```python
from build123d import *

# Parameters (mm, degrees)
SKETCH1_R             = 19.75
BOSS_EXTRUDE1_DEPTH   = 5
CUT_EXTRUDE1_DEPTH    = 4.2
F_8_CLEARANCE_HOLE1_D = 4.4958
CUT_EXTRUDE2_DEPTH    = 10


with BuildPart() as part:
    # Sketch1 → Boss-Extrude1 (new, symmetric)
    with BuildSketch(Plane(origin=(0, 0, 0), x_dir=(1, 0, 0), z_dir=(0, 1, 0))):
        with Locations(Location((0, 0, 0), (0, 0, 270))):
            Circle(SKETCH1_R)
    extrude(amount=BOSS_EXTRUDE1_DEPTH, both=True)

    # Sketch2 → Cut-Extrude1 (cut)
    with BuildSketch(Plane(origin=(0, 5, 0), x_dir=(1, 0, 0), z_dir=(0, 1, 0))):
        Polygon((-8.9, -3.637306696), (-6.8, 0), (-8.9, 3.637306696), (-13.1, 3.637306696), (-15.2, 0), (-13.1, -3.637306696), align=None)
        Polygon((13.1, -3.637306696), (8.9, -3.637306696), (6.8, 0), (8.9, 3.637306696), (13.1, 3.637306696), (15.2, 0), align=None)
    extrude(amount=-CUT_EXTRUDE1_DEPTH, mode=Mode.SUBTRACT)

    # 8 Clearance Hole1 (through all)
    with Locations(Plane(origin=(0, 0.8, 0), x_dir=(1, 0, 0), z_dir=(0, 1, 0))):
        with Locations((-11, 0), (11, 0)):
            Hole(F_8_CLEARANCE_HOLE1_D / 2)

    # Sketch6 → Cut-Extrude2 (cut)
    with BuildSketch(Plane(origin=(0, 5, 0), x_dir=(1, 0, 0), z_dir=(0, 1, 0))):
        with BuildLine():
            ThreePointArc((16.403124702, 11), (0, 19.75), (-16.403124702, 11))
            Line((-16.403124702, 11), (16.403124702, 11))
        make_face()
        with BuildLine():
            Line((16.403124702, -11), (-16.403124702, -11))
            ThreePointArc((-16.403124702, -11), (0, -19.75), (16.403124702, -11))
        make_face()
    extrude(amount=-CUT_EXTRUDE2_DEPTH, mode=Mode.SUBTRACT)


solid = part.part
```
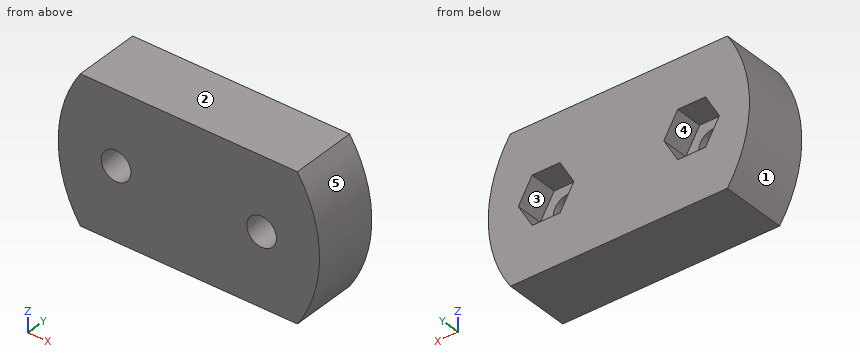
Can you work these out from the model? Positions are in its coordinate system, mm. Face numbers are marked on the shaded views. A direction names the side the tool comes from. Coordinates: 2 decimals unless noted, no trailing zeros. Write each loop counter-clockwise with the first axis right and the second up, starting at its lowest first coordinate (ties: lowest second). Pieces come first, ordered by that corner, then holes. Notation, with made-up numbers: (19, 24) - (39, 24) arc R17 cw to (39, 50) - close; hole circle Ø4 at (57, 42). An arc over 180 degrees is marked (long way). Return JSON: item names as keys, results as strings.
Q1. Thinking about a two-plate mould opening in Z: for the marked faces 1, 2 and 3, which applies, +Z half, -Z half, draft (parallel to the pull), parting line (faces both ways), or undercut?
Computed values:
{"face 1": "parting line", "face 2": "+Z half", "face 3": "undercut"}
Q2. I'm going to push flat-ended pins straight in: pin 1 Ø5 at (x, z) = (11, 0) entering from +Y; pin 2 Ø6 at (x, z) = (-11, 0) entering from -Y; pin 3 Ø2 at (y, z) = (0, 5.5) entering from +X; pin 4 Ø4 at (y, z) = (0.5, 3) entering from +X. Where does each tip first touch, or does it pass through?
Computed values:
{"pin 1": "stops at y = 0.8", "pin 2": "stops at y = -5", "pin 3": "stops at x = 19.23", "pin 4": "stops at x = 19.72"}
Q3. On a 3-axis mill with a long thin cutter (end or side, diameter ignored), from which of +Z, -Z, +X, -X, +Y, -Y can I reach the whole of each face in a straight line? I mean the marked faces 4 and 5. Say none if no direction works.
Computed values:
{"face 4": "+Y", "face 5": "+X, +Y, -Y"}
Q4. If we section it at D-D (z = 3.25): Please give me the cut outline in (x, y), then the cut area to 3 significant figures.
Computed values:
{"outline": "(-19.48, -5) - (19.48, -5) - (19.48, 5) - (13.32, 5) - (13.32, 0.8) - (8.68, 0.8) - (8.68, 5) - (-8.68, 5) - (-8.68, 0.8) - (-13.32, 0.8) - (-13.32, 5) - (-19.48, 5) - close", "area": "351 mm2"}
Q5. If we section it at B-B (z = -0.5): Please give me the cut outline in (x, y).
Computed values:
{"outline": "(-19.74, -5) - (-13.19, -5) - (-13.19, 0.8) - (-14.91, 0.8) - (-14.91, 5) - (-19.74, 5) - close; (-8.81, -5) - (8.81, -5) - (8.81, 0.8) - (7.09, 0.8) - (7.09, 5) - (-7.09, 5) - (-7.09, 0.8) - (-8.81, 0.8) - close; (13.19, -5) - (19.74, -5) - (19.74, 5) - (14.91, 5) - (14.91, 0.8) - (13.19, 0.8) - close"}
Q6. If we section it at C-C (y = 3.75): Please give me the cut outline in (x, z), then the cut area to 3 significant figures.
Computed values:
{"outline": "(-16.4, -11) - (16.4, -11) arc R19.75 ccw to (16.4, 11) - (-16.4, 11) arc R19.75 ccw to start; hole (-15.2, 0) - (-13.1, -3.64) - (-8.9, -3.64) - (-6.8, 0) - (-8.9, 3.64) - (-13.1, 3.64) - close; hole (6.8, 0) - (8.9, -3.64) - (13.1, -3.64) - (15.2, 0) - (13.1, 3.64) - (8.9, 3.64) - close", "area": "730 mm2"}
Q7. If we section it at A-A (x = -11): Please give me the cut outline in (y, z), then the cut area to 3 significant figures.
Computed values:
{"outline": "(-5, -11) - (5, -11) - (5, -3.64) - (0.8, -3.64) - (0.8, -2.25) - (-5, -2.25) - close; (-5, 2.25) - (0.8, 2.25) - (0.8, 3.64) - (5, 3.64) - (5, 11) - (-5, 11) - close", "area": "163 mm2"}
Q8. Please list where these lines run through material, in increasing order: L1, parallel to Z at x = 11, y = -1; L2, parallel to X at y = 1, z = 1; L3, parallel to X at y = -3, z = 0.25. Write a range as from..to.
Computed values:
{"L1": "z = -11..-2.25, 2.25..11", "L2": "x = -19.72..-14.62, -7.38..7.38, 14.62..19.72", "L3": "x = -19.75..-13.23, -8.77..8.77, 13.23..19.75"}
